Autodesk Inventor part; units mm, degrees
ref_plane "YZ Plane" through (0, 0, 0) normal (1, 0, 0) x (0, 1, 0)
ref_plane "XZ Plane" through (0, 0, 0) normal (0, 1, 0) x (-1, 0, 0)
ref_plane "XY Plane" through (0, 0, 0) normal (0, 0, 1) x (1, 0, 0)
sketch "Sketch1" plane through (0, 0, 0) normal (1, 0, 0) x (0, 1, 0)
  line L0 (0, 0) -> (2, 0)
  line L1 (0, 0) -> (0, -18)
  line L2 (2, -20) -> (20, -20)
  line L3 (20, -20) -> (20, -18)
  line L4 (20, -18) -> (2, -18)
  line L5 (2, 0) -> (2, -18)
  arc A0 (0, -18) -> (2, -20) centre (2, -18) ccw
  point P0 (0, -20)
  dimension "d0" = 2
  dimension "d1" = 20
  dimension "d2" = 20
  dimension "d3" = 2
  dimension "d4" = 2
extrude "Extrusion1" add sketch "Sketch1" along normal blind 16
fillet "Fillet2" radius 8 4 edges at (16, 20, -19) (0, 20, -19) (0, 1, 0) (16, 1, 0)
sketch "Sketch2" plane through (0, 2, -18) normal (0, 0, 1) x (1, 0, 0)
  line L0 (0, 0) -> (0, 10)
  line L1 (0, 0) -> (16, 0)
  line L2 (16, 10) -> (16, 0)
  arc A0 (16, 10) -> (0, 10) centre (8, 10) ccw
  line L3 (0, 0) -> (16, 0)
  point P0 (0, -2)
hole "Hole1" at (8, 12, -18) direction (0, 0, -1) diameter 4.2 end through all countersink diameter 6 countersink angle 90
sketch "Sketch4" plane through (0, 2, -18) normal (0, 1, 0) x (1, 0, 0)
  arc A0 (0, -10) -> (16, -10) centre (8, -10) ccw
  line L0 (16, 0) -> (16, -10)
  line L1 (0, 0) -> (16, 0)
  line L2 (0, -10) -> (0, 0)
  point P0 (0, -18)
hole "Hole3" at (8, 2, -8) direction (0, -1, 0) diameter 4.2 end through all countersink diameter 6 countersink angle 90
properties part number "MellewellCornerBrace"
Could you check a few things on this model? Use its own coordinates, in mm. A direction names the side the tool comes from. Give positions to 0.01 mm unless a question says otherwise; leave off trailing zeros. Order: outer loops, then holes, each group sorted by start corner. A loop starts at its lowest first (then second) coordinate and runs counter-clockwise, first axis right, second up. Notation, with made-up numbers: (86.5, 39.5) - (132.5, 39.5) arc R34 ccw to (132.5, 74.5) - close; hole circle Ø5 at (48, 27). An arc over 180 degrees is marked (long way). One line per question, with ' | ' between items. Start each with the question number.
Item 1: I want a section at D-D on x = 7.25. Give the number of separate pieces and of enclosed holes in the cut face, then the cut area to 3 significant figures.
Item 2: I'm going to push flat-ended pins straight in: pin 1 Ø4 at (y, z) = (5.5, -4) entering from +X; pin 2 Ø5 at (x, y) = (8.5, 10.5) entering from +Z. Where does each tip first touch, or does it pass through?
Item 3: I want a section at B-B on y = 8.5. Write out the boundary of the cut face in (x, z), then the cut area to 3 significant figures.
Item 4: I need wall thicknesses on probe 1 along X at (y, z) = (12, -19.55); probe 2 along Y at (x, z) = (10.5, -17.5); probe 3 along Z at (x, y) = (14, 7.25). Which ranges of each line are inside material? Lowest first, please. Write a range as [from, to].
Item 5: For faces 1 (the flat face through (10, 2, -11)), 2 (the cylindrical face through (13.719, 17.594, -18.986)), which set-ups out of +Z, -Z, +X, -X, +Y, -Y let a thin tool reach every point of the face, with its end or its side?
Item 6: Thinking about a two-plate mould opening in Z: for faces 3 (the cylindrical face through (5.918, 0.542, -8.273)), 4 (the cylindrical face through (2.406, 17.719, -18.986)), 5 (the cylindrical face through (7.89, 0.6, -19.43)), which applies, pulls with the +Z half, pulls with the -Z half, needs draft (parallel to the pull), parting line crosses it, or undercut?
Item 7: I want a section at A-A on x = 1. Write out the boundary of the cut face in (y, z), then the cut area to 3 significant figures.
Item 8: I want a section at C-C on z = -16.75. Write out the boundary of the cut face in (x, y), then the cut area to 3 significant figures.
Verdict:
1) separate pieces: 3 | enclosed holes: 0 | area: 57.6 mm^2
2) pin 1: through | pin 2: z = -18
3) outline: (0, -20) - (16, -20) - (16, -18) - (0, -18) - close | area: 32.0 mm^2
4) probe 1: [0, 5.9], [10.1, 16] | probe 2: [0, 2] | probe 3: [-20, -18]
5) face 1: +Z, +X, -X, +Y | face 2: +Z, -Z, +X, +Y
6) face 3: undercut | face 4: needs draft | face 5: pulls with the -Z half
7) outline: (0, -18) arc R2 ccw to (2, -20) - (15.87, -20) - (15.87, -18) - (2, -18) - (2, -4.13) - (0, -4.13) - close | area: 58.6 mm^2
8) outline: (0, 0) - (16, 0) - (16, 2) - (0, 2) - close | area: 32.0 mm^2
